```python
from build123d import *

# Parameters (mm, degrees)
SKETCH_R   = 3
SKETCH_R_2 = 8
PAD_DEPTH  = 25


with BuildPart() as part:
    # Sketch → Pad (new body)
    with BuildSketch(Plane.XY):
        with BuildLine():
            ThreePointArc((-46.2, -24.936118), (0, -52.5), (46.2, -24.936118))
            ThreePointArc((46.2, -24.936118), (47.54304, -21.485748), (48, -17.811513))
            Line((48, 17.811513), (48, -17.811513))
            ThreePointArc((48, 17.811513), (47.54304, 21.485748), (46.2, 24.936118))
            ThreePointArc((46.2, 24.936118), (0, 52.5), (-46.2, 24.936118))
            ThreePointArc((-46.2, 24.936118), (-47.54304, 21.485748), (-48, 17.811513))
            Line((-48, 17.811513), (-48, -17.811513))
            ThreePointArc((-48, -17.811513), (-47.54304, -21.485748), (-46.2, -24.936118))
        make_face()
        with Locations((22.273864, 22.273864)):
            Circle(SKETCH_R, mode=Mode.SUBTRACT)
        with Locations((0, 31.5)):
            Circle(SKETCH_R, mode=Mode.SUBTRACT)
        with Locations((31.5, 0)):
            Circle(SKETCH_R, mode=Mode.SUBTRACT)
        with Locations((0, -31.5)):
            Circle(SKETCH_R, mode=Mode.SUBTRACT)
        with Locations((-22.273864, -22.273864)):
            Circle(SKETCH_R, mode=Mode.SUBTRACT)
        with Locations((-31.5, 0)):
            Circle(SKETCH_R, mode=Mode.SUBTRACT)
        with Locations((-22.273864, 22.273864)):
            Circle(SKETCH_R, mode=Mode.SUBTRACT)
        with Locations((22.273864, -22.273864)):
            Circle(SKETCH_R, mode=Mode.SUBTRACT)
        with Locations((-17.029413, 41.112639)):
            Circle(SKETCH_R, mode=Mode.SUBTRACT)
        with Locations((17.029413, 41.112639)):
            Circle(SKETCH_R, mode=Mode.SUBTRACT)
        with Locations((41.112639, 17.029413)):
            Circle(SKETCH_R, mode=Mode.SUBTRACT)
        with Locations((41.112639, -17.029413)):
            Circle(SKETCH_R, mode=Mode.SUBTRACT)
        with Locations((17.029413, -41.112639)):
            Circle(SKETCH_R, mode=Mode.SUBTRACT)
        with Locations((-17.029413, -41.112639)):
            Circle(SKETCH_R, mode=Mode.SUBTRACT)
        with Locations((-41.112639, -17.029413)):
            Circle(SKETCH_R, mode=Mode.SUBTRACT)
        with Locations((-41.112639, 17.029413)):
            Circle(SKETCH_R, mode=Mode.SUBTRACT)
        Circle(SKETCH_R_2, mode=Mode.SUBTRACT)
    extrude(amount=PAD_DEPTH)


solid = part.part
```
Geometry: final body of the model. Coordinates: model frame, mm. Coordinates: 2 decimals unless noted, no trailing zeros. Order: outer loops, then holes, each group sorted by start corner. A loop starts at its lowest first (then second) coordinate and runs counter-clockwise, first axis right, second up.
Item 1: Contact query for flat-ended pins moving along their axis: P1, Ø5, axis at x = -17.03, y = 41.11, coming from the -Z side; P2, Ø10, axis at x = 36.5, z = 17, coming from the -Y side; P3, Ø5, axis at y = -38.5, z = 2.5, coming from the +X side; P4, Ø2, axis at y = -26.5, z = 4.5, coming from the +X side. Output: stop coordinate, or through.
Answer:
P1: passes through
P2: stops at y = -42
P3: stops at x = 38.21
P4: stops at x = 45.89
Item 2: Material intervals for line 1 along Y through (x, z) = (-25, 6.5); line 2 along Y through (x, z) = (-20.5, 18.5); line 3 along X through (y, z) = (-22.5, 2.75), sorted ascending.
Answer:
line 1: y = -46.17 to -23.53, -21.02 to 21.02, 23.53 to 46.17
line 2: y = -48.33 to -24.69, -19.85 to 19.85, 24.69 to 48.33
line 3: x = -47.25 to -25.27, -19.28 to 19.28, 25.27 to 47.25
Item 3: Section query A-A (x = 0). Output: boundary loops of the cut face in (y, z), then the cut area to 4 significant figures.
Answer:
outline: (-52.5, 0) - (-34.5, 0) - (-34.5, 25) - (-52.5, 25) - close; (-28.5, 0) - (-8, 0) - (-8, 25) - (-28.5, 25) - close; (8, 0) - (28.5, 0) - (28.5, 25) - (8, 25) - close; (34.5, 0) - (52.5, 0) - (52.5, 25) - (34.5, 25) - close
area: 1,925 mm2
Item 4: Section query B-B (y = 31.5). Output: boundary loops of the cut face in (x, z), then the cut area to 3 significant figures.
Answer:
outline: (-42, 0) - (-3, 0) - (-3, 25) - (-42, 25) - close; (3, 0) - (42, 0) - (42, 25) - (3, 25) - close
area: 1,950 mm2
Item 5: Section query D-D (z = 2). State how many separate pieces and enclosed holes the cut face has, then the cut area to 3 significant figures.
Answer:
separate pieces: 1
enclosed holes: 17
area: 7,740 mm2
Item 6: Draft query along X for faces 1 (the face through (47.556, 21.435, 12.325)), 2 (the face through (-24.655, -24.099, 12.325)), 3 (the face through (-48, 0, 12)). Return one class per face: released by +X, released by -X, zero draft, split by the parting line, or undercut.
Answer:
face 1: released by +X
face 2: undercut
face 3: released by -X
